```python
from build123d import *

# Parameters (mm, degrees)
SKETCH_1_W          = 109
SKETCH_1_H          = 109
SKETCH_1_R          = 1.6
EXTRUDE_2_DEPTH     = 5
FILLET_1_R          = 3
SKETCH_2_R          = 3
CUT_EXTRUDE_1_DEPTH = 3.3


with BuildPart() as part:
    # 草图1 → 凸台-拉伸2 (new body)
    with BuildSketch(Plane(origin=(0, 0, 0), x_dir=(1, 0, 0), z_dir=(0, 1, 0))):
        with Locations((54.5, 54.5)):
            Rectangle(SKETCH_1_W, SKETCH_1_H)
        with Locations((14.5, 94.5)):
            Circle(SKETCH_1_R, mode=Mode.SUBTRACT)
        with Locations((94.5, 94.5)):
            Circle(SKETCH_1_R, mode=Mode.SUBTRACT)
        with Locations((94.5, 14.5)):
            Circle(SKETCH_1_R, mode=Mode.SUBTRACT)
        with Locations((14.5, 14.5)):
            Circle(SKETCH_1_R, mode=Mode.SUBTRACT)
        Polygon((14.5, 87.428932188), (47.428932188, 54.5), (14.5, 21.571067812), align=None, mode=Mode.SUBTRACT)
        Polygon((21.571067812, 94.5), (87.428932188, 94.5), (54.5, 61.571067812), align=None, mode=Mode.SUBTRACT)
        Polygon((94.5, 87.428932188), (94.5, 21.571067812), (61.571067812, 54.5), align=None, mode=Mode.SUBTRACT)
        Polygon((87.428932188, 14.5), (21.571067812, 14.5), (54.5, 47.428932188), align=None, mode=Mode.SUBTRACT)
    extrude(amount=EXTRUDE_2_DEPTH)

    # 圆角1
    fillet_1_edges = [part.edges().sort_by_distance(p)[0] for p in [
        (14.5, 2.5, -87.428932188),
        (14.5, 2.5, -21.571067812),
        (47.428932188, 2.5, -54.5),
        (54.5, 2.5, -61.571067812),
        (87.428932188, 2.5, -94.5),
        (21.571067812, 2.5, -94.5),
        (61.571067812, 2.5, -54.5),
        (94.5, 2.5, -21.571067812),
        (94.5, 2.5, -87.428932188),
        (54.5, 2.5, -47.428932188),
        (21.571067812, 2.5, -14.5),
        (87.428932188, 2.5, -14.5),
        (0, 2.5, -109),
        (109, 2.5, -109),
        (109, 2.5, 0),
        (0, 2.5, 0),
    ]]
    fillet(fillet_1_edges, radius=FILLET_1_R)

    # 草图2 → 切除-拉伸1 (cut)
    with BuildSketch(Plane.XZ):
        with Locations((14.5, -14.5)):
            Circle(SKETCH_2_R)
        with Locations((94.5, -14.5)):
            Circle(SKETCH_2_R)
        with Locations((94.5, -94.5)):
            Circle(SKETCH_2_R)
        with Locations((14.5, -94.5)):
            Circle(SKETCH_2_R)
    extrude(amount=-CUT_EXTRUDE_1_DEPTH, mode=Mode.SUBTRACT)


solid = part.part
```
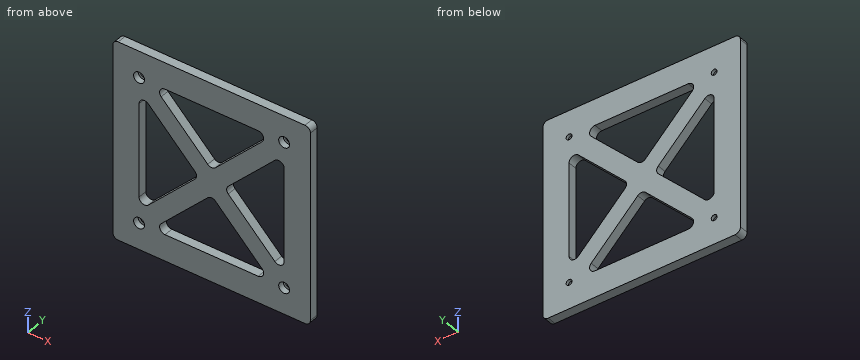
Build history of the part. All positions in model axes, mm. Coordinates: 2 decimals unless noted, no trailing zeros. Order: outer loops, then holes, each group sorted by start corner. A loop starts at its lowest first (then second) coordinate and runs counter-clockwise, first axis right, second up. Notation, with made-up numbers: M 7,13 L 41,13 A15 cw 41,31 Z; hole C 33,78.5 d1. An arc over 180 degrees is marked long. One line per question, with ' | ' between items. Start each with the question number.
1. Cut at B-B (x = 86.5). Write the cut outline in (y, z), plus the area to 3 significant figures.
2. Cut at A-A (z = -88). Write the cut outline in (x, y), plus the area to 3 significant figures.
3. Cut at D-D (z = -73.5). Write the cut outline in (x, y), plus the area to 3 significant figures.
4. Flat gauge pins, fed straight in: P1, Ø1.9, axis at x = 94.5, z = -94.5, coming from the +Y side; P2, Ø3, axis at x = 14.5, z = -95, coming from the -Y side. Where does each tip first touch, or does it go through?
5. Wall check: line 1 along Z through (x, y) = (54.5, 2.9); line 2 along X through (y, z) = (4, -52.5); line 3 along X through (y, z) = (2.85, -66.5). Give the ranges that are in metal, low to high. Write a range as [from, to].
6. Cut at C-C (y = 1.4). Count the separate pieces of the cut face and the enclosed holes in it, plus the area to 3 significant figures.
The answers:
1) outline: M 0,-109 L 5,-109 L 5,-79.43 L 0,-79.43 Z; M 0,-29.57 L 5,-29.57 L 5,0 L 0,0 Z | area: 296 mm2
2) outline: M 0,0 L 28.07,0 L 28.07,5 L 0,5 Z; M 80.93,0 L 109,0 L 109,5 L 80.93,5 Z | area: 281 mm2
3) outline: M 0,0 L 14.5,0 L 14.5,5 L 0,5 Z; M 28.43,0 L 42.57,0 L 42.57,5 L 28.43,5 Z; M 66.43,0 L 80.57,0 L 80.57,5 L 66.43,5 Z; M 94.5,0 L 109,0 L 109,5 L 94.5,5 Z | area: 286 mm2
4) P1: passes through | P2: stops at y = 3.3
5) line 1: z = [-109, -94.5], [-62.81, -46.19], [-14.5, 0] | line 2: x = [0, 14.5], [45.42, 63.58], [94.5, 109] | line 3: x = [0, 14.5], [35.43, 49.57], [59.43, 73.57], [94.5, 109]
6) separate pieces: 1 | enclosed holes: 8 | area: 7,520 mm2
